Work out the finished part from the listing and answer in its coordinate system (mm). A direction names the side the tool comes from. Coordinates: 2 decimals unless noted, no trailing zeros. Order: outer loops, then holes, each group sorted by start corner. A loop starts at its lowest first (then second) coordinate and runs counter-clockwise, first axis right, second up.
1. The part is cut by section A-A, the plane y = 0.85. Give the vertices of the cut face in (x, z) (3 decimals), then the cut area to 3 significant figures.
2. A flat-ended cylindrical pin translates along its axis: pin 1 Ø3.5 at (x, z) = (4, -7) entering from -Y. Find the tip coordinate at first contact, or state that the pin passes through.
3. A tool of negligible diameter and unlimited length cuts with its end or side. For faces 1 (the flat face through (5, 1.905, -9)), 2 (the flat face through (6, 1, 0)), from which of +Z, -Z, +X, -X, +Y, -Y can it reach the whole face along a straight path? Write none if from no direction.
4. The part is cut by section C-C, the plane z = -2.5. Give the vertices of the cut face in (x, y) (3 decimals), then the cut area to 3 significant figures.
5. The part is cut by section D-D, the plane x = 9.75. Give the vertices of the cut face in (y, z) (3 decimals), then the cut area to 3 significant figures.
6. Find the intervals of material crossed by probe 1 along Z at (x, y) = (11, 0.5) (3 decimals); probe 2 along X at (y, z) = (1.1, -10.5) (3 decimals); probe 3 along Z at (x, y) = (5.5, 1) (3 decimals), in increasing order.
7. Determine the mould class of faces 3 (the flat face through (0, 1, -6)), 4 (the flat face through (12.7, 1, -6)), 5 (the flat face through (6, 0, -6)), 6 (the cylindrical face through (8.83, 0.97, -6.9)) for opening direction X: +X half, -X half, draft (parallel to the pull), parting line (faces both ways), or undercut.
```python
from build123d import *

# Parameters (mm, degrees)
SKETCH1_W           = 12.7
SKETCH1_H           = 12.7
BOSS_EXTRUDE1_DEPTH = 2.54
FILLET1_R           = 0.635
SHELL1_START        = 0.635
SHELL1_OUTLINE_W    = 1.905
SHELL1_OUTLINE_H    = 11.43
SHELL1_DEPTH        = 11.43
SKETCH2_R           = 2.54
BOSS_EXTRUDE2_DEPTH = 1.905
BOSS_EXTRUDE3_DEPTH = 0.00254


# Read off the part's stored shape, not the designer's step: Shell1
with BuildPart() as part:
    # Sketch1 → Boss-Extrude1 (new body)
    with BuildSketch(Plane(origin=(0, 0, 0), x_dir=(1, 0, 0), z_dir=(0, 1, 0))):
        with Locations((6.35, 6.35)):
            Rectangle(SKETCH1_W, SKETCH1_H)
    extrude(amount=BOSS_EXTRUDE1_DEPTH)

    # Fillet1
    fillet1_edges = [part.edges().sort_by_distance(p)[0] for p in [
        (0, 1.27, -12.7),
        (12.7, 1.27, -12.7),
        (12.7, 1.27, 0),
        (0, 1.27, 0),
    ]]
    fillet(fillet1_edges, radius=FILLET1_R)

    # Shell1 outline → Shell1 (cut)
    with BuildSketch(Plane.YZ.offset(SHELL1_START)):
        with Locations((0.9525, -6.35)):
            Rectangle(SHELL1_OUTLINE_W, SHELL1_OUTLINE_H)
    extrude(amount=SHELL1_DEPTH, mode=Mode.SUBTRACT)

    # Sketch2 → Boss-Extrude2 (add)
    with BuildSketch(Plane(origin=(0, 1.905, 0), x_dir=(-1, 0, 0), z_dir=(0, -1, 0))):
        with Locations(Location((-6.35, 6.35, 0), (0, 0, 270))):
            Circle(SKETCH2_R)
    extrude(amount=BOSS_EXTRUDE2_DEPTH)

    # Sketch3 → Boss-Extrude3 (add)
    with BuildSketch(Plane(origin=(0, 2.54, 0), x_dir=(1, 0, 0), z_dir=(0, 1, 0))):
        Polygon((5.573346154, 8.001), (7.120141026, 8.001), (7.120141026, 7.431128205), (6.143217949, 7.431128205), (6.143217949, 6.820551282), (7.120141026, 6.820551282), (7.120141026, 6.250679487), (6.143217949, 6.250679487), (6.143217949, 4.826), (5.573346154, 4.826), align=None)
    extrude(amount=BOSS_EXTRUDE3_DEPTH)


solid = part.part
```
Geometry says:
1. outline: (0, -12.065) arc R0.635 ccw to (0.635, -12.7) - (12.065, -12.7) arc R0.635 ccw to (12.7, -12.065) - (12.7, -0.635) arc R0.635 ccw to (12.065, 0) - (0.635, 0) arc R0.635 ccw to (0, -0.635) - close; circle Ø5.08 at (6.35, -6.35); hole (0.635, -12.065) - (12.065, -12.065) - (12.065, -0.635) - (0.635, -0.635) - close
1. area: 50.6 mm2
2. pin 1: stops at y = 0
3. face 1: -Y
3. face 2: +Z, +X, -X, +Y, -Y
4. outline: (0, 0) - (0.635, 0) - (0.635, 1.905) - (12.065, 1.905) - (12.065, 0) - (12.7, 0) - (12.7, 2.54) - (0, 2.54) - close
4. area: 10.5 mm2
5. outline: (0, -12.7) - (2.54, -12.7) - (2.54, 0) - (0, 0) - (0, -0.635) - (1.905, -0.635) - (1.905, -12.065) - (0, -12.065) - close
5. area: 10.5 mm2
6. probe 1: z = -12.7 to -12.065, -0.635 to 0
6. probe 2: x = 0 to 0.635, 12.065 to 12.7
6. probe 3: z = -12.7 to -12.065, -8.744 to -3.956, -0.635 to 0
7. face 3: -X half
7. face 4: +X half
7. face 5: draft
7. face 6: undercut
